The drawing under review shows one solid part. Ordinate dimensions are in mm from its lowest x, y, z. Coordinates: 2 decimals unless noted, no trailing zeros. Write each loop counter-clockwise with the first axis right and the second up, starting at its lowest first coordinate (ties: lowest second). Pieces come first, ordered by that corner, then holes.
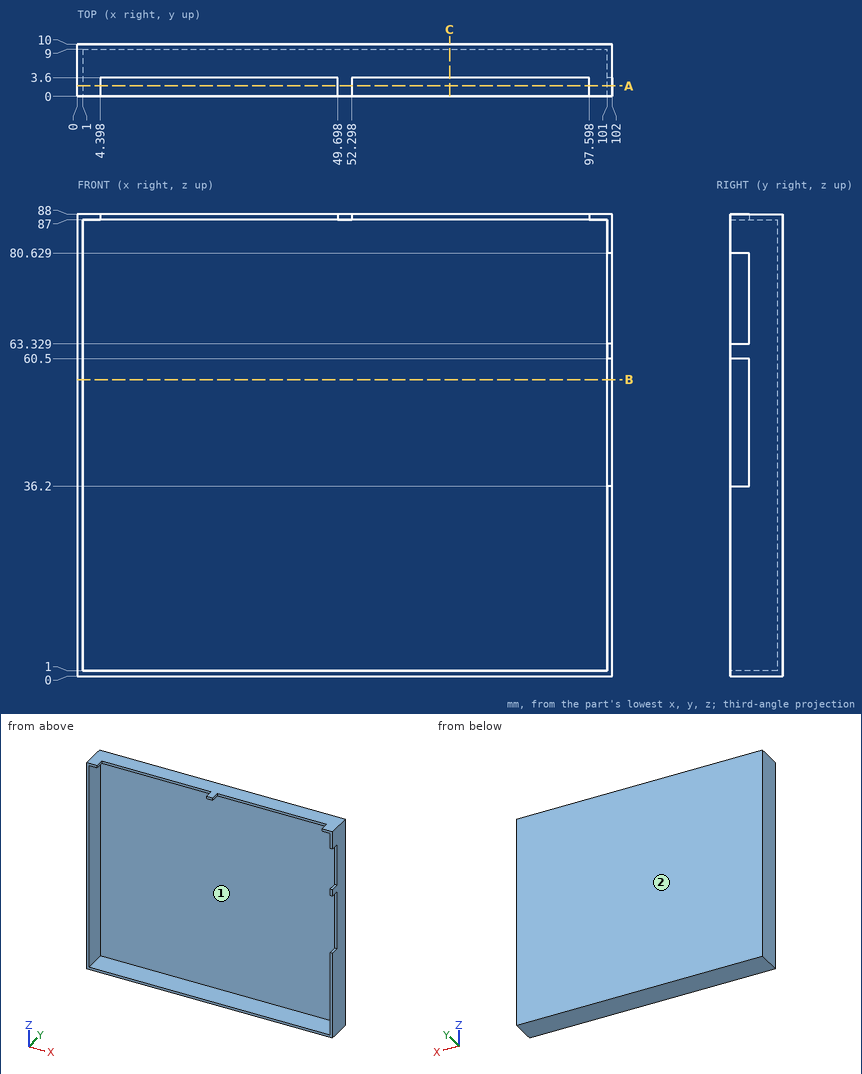
Q1. Add section C-C (x = 71). State the section outline as (y, z) points, then the cut area to 3 significant figures.
Ans:
outline: (0, 0) - (10, 0) - (10, 88) - (3.6, 88) - (3.6, 87) - (9, 87) - (9, 1) - (0, 1) - close
area: 102 mm2
Q2. For probe 1 along Z at (x, y) = (7.5, 8); probe 2 along X at (y, z) = (7, 61); probe 3 along Y at (x, z) = (87, 27), list the stretches that pass through material, from the lowest coordinate up.
Ans:
probe 1: z = 0 to 1, 87 to 88
probe 2: x = 0 to 1, 101 to 102
probe 3: y = 9 to 10
Q3. Add section B-B (z = 56.5). State the section outline as (x, y) points, then the cut area to 3 significant figures.
Ans:
outline: (0, 0) - (1, 0) - (1, 9) - (101, 9) - (101, 3.6) - (102, 3.6) - (102, 10) - (0, 10) - close
area: 116 mm2
Q4. Clearance check with flat-ended pins moving along their axes: pin 1 Ø2 at (x, z) = (17, 72) entering from -Y; pin 2 Ø0.8 at (x, z) = (32.5, 87.5) entering from -Y. State where each tip first meets the part, or that it passes through.
Ans:
pin 1: stops at y = 9
pin 2: stops at y = 3.6
Q5. Add section A-A (y = 2). State the section outline as (x, z) points.
Ans:
outline: (0, 0) - (102, 0) - (102, 36.2) - (101, 36.2) - (101, 1) - (1, 1) - (1, 87) - (4.4, 87) - (4.4, 88) - (0, 88) - close; (49.7, 87) - (52.3, 87) - (52.3, 88) - (49.7, 88) - close; (97.6, 87) - (101, 87) - (101, 80.63) - (102, 80.63) - (102, 88) - (97.6, 88) - close; (101, 60.5) - (102, 60.5) - (102, 63.33) - (101, 63.33) - close
Q6. Draft analysis for pull direction Z (two halves, no side actions). For the marked faces 1 and 2, state which applies: +Z half, -Z half, draft (parallel to the pull), parting line (faces both ways), or undercut.
Ans:
face 1: undercut
face 2: draft
